Geometry check sheet. Reference: drawing and pictorial views, mm from the part's lowest x, y, z. A direction names the side the tool comes from. Give positions to 0.01 mm unless a question says otherwise; leave off trailing zeros. Order: outer loops, then holes, each group sorted by start corner. A loop starts at its lowest first (then second) coordinate and runs counter-clockwise, first axis right, second up. Notation, with made-up numbers: M 84.25,39.25 L 103.25,39.25 A35 ccw 103.25,73.25 Z; hole C 75.5,6 d7. An arc over 180 degrees is marked long. Use CSV: the item, a comma, the result in double quotes. Start each with the question number.
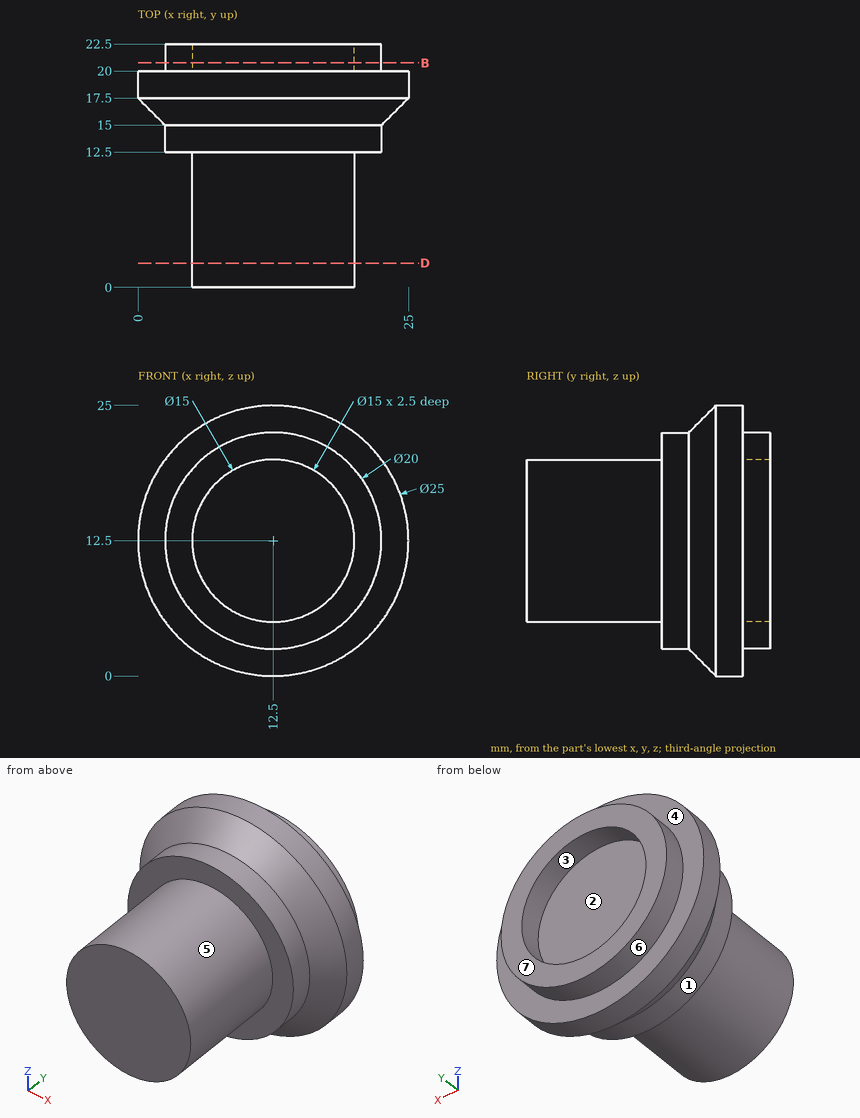
(1) Go/stop test with flat-tipped pins: P1, Ø12, axis at x = 12.5, z = 12.5, coming from the +Y side; P2, Ø4, axis at y = 20, z = 19, coming from the -X side; P3, Ø1.5, axis at x = 4.5, y = 19.5, coming from the -Z side; P4, Ø1, axis at x = 7.5, z = 21.5, coming from the +Y side. Record where each tip stops, or that it passes through.
(2) Draft check along Z on the marked faces 1, 2, 3 and 4. Enter one of: +Z half, -Z half, draft (parallel to the pull), parting line (faces both ways), or undercut.
(3) Thickness scan on line 1 (Z direction, x = 12.5, y = 21.2); line 2 (Y direction, x = 7, z = 17.75); line 3 (Y direction, x = 14.75, z = 12). Record the ranges inside material, lowest first.
(4) Sectioned sample at D-D on y = 2.25. Record the cut outline in (x, z).
(5) Access from +Z, -Z, +X, -X, +Y, -Y to the whole of each face (thin tool, end or side, straight path). Record for the marked faces 5, 6 and 7.
(6) Sectioned sample at B-B on y = 20.75. Record the cut outline in (x, z).
Responses:
1,P1,"y = 20"
1,P2,"x = 0.84"
1,P3,"z = 2.32"
1,P4,"y = 22.5"
2,face 1,"parting line"
2,face 2,"undercut"
2,face 3,"undercut"
2,face 4,"draft"
3,line 1,"2.5 to 5, 20 to 22.5"
3,line 2,"12.5 to 22.5"
3,line 3,"0 to 20"
4,outline,"C 12.5,12.5 d15"
5,face 5,"-Y"
5,face 6,"+Y"
5,face 7,"+Z, -Z, +X, -X, +Y"
6,outline,"C 12.5,12.5 d20; hole C 12.5,12.5 d15"
